from build123d import *

# Parameters (mm, degrees)
SZKIC1_R                    = 5
SZKIC1_R_2                  = 21.5
DODANIE_WYCI_GNI_CIE1_DEPTH = 3
DODANIE_WYCI_GNI_CIE2_DEPTH = 3


with BuildPart() as part:
    # Szkic1 → Dodanie-wyciągnięcie1 (new body)
    with BuildSketch(Plane.XY):
        with BuildLine():
            ThreePointArc((10, 35), (0, 45), (-10, 35))
            ThreePointArc((-10, 35), (-17.32233047, 17.32233047), (-35, 10))
            ThreePointArc((-35, 10), (-45, 0), (-35, -10))
            ThreePointArc((-35, -10), (-17.32233047, -17.32233047), (-10, -35))
            ThreePointArc((-10, -35), (0, -45), (10, -35))
            ThreePointArc((10, -35), (17.32233047, -17.32233047), (35, -10))
            ThreePointArc((35, -10), (45, 0), (35, 10))
            ThreePointArc((35, 10), (17.32233047, 17.32233047), (10, 35))
        make_face()
        with Locations((0, 35)):
            Circle(SZKIC1_R, mode=Mode.SUBTRACT)
        Circle(SZKIC1_R_2, mode=Mode.SUBTRACT)
        with Locations((35, 0)):
            Circle(SZKIC1_R, mode=Mode.SUBTRACT)
        with Locations((0, -35)):
            Circle(SZKIC1_R, mode=Mode.SUBTRACT)
        with Locations((-35, 0)):
            Circle(SZKIC1_R, mode=Mode.SUBTRACT)
    extrude(amount=DODANIE_WYCI_GNI_CIE1_DEPTH)

    # Szkic2 → Dodanie-wyciągnięcie2 (add)
    with BuildSketch(Plane.XY):
        with BuildLine():
            Line((27.599747415, 5.722247038), (37.016747674, 9.794525452))
            ThreePointArc((37.016747674, 9.794525452), (19.32662719, 19.32662719), (9.794525452, 37.016747674))
            Line((9.794525452, 37.016747674), (8.161162093, 24.785340239))
            Line((8.161162093, 24.785340239), (27.599747415, 5.722247038))
        make_face()
        with BuildLine():
            Line((-5.468778256, 25.979107706), (-9.794525452, 37.016747674))
            ThreePointArc((-9.794525452, 37.016747674), (-19.32662719, 19.32662719), (-37.016747674, 9.794525452))
            Line((-37.016747674, 9.794525452), (-28.775607604, 5.722247038))
            Line((-28.775607604, 5.722247038), (-5.468778256, 25.979107706))
        make_face()
        with BuildLine():
            ThreePointArc((-9.794525452, -37.016747674), (-19.32662719, -19.32662719), (-37.016747674, -9.794525452))
            Line((-37.016747674, -9.794525452), (-27.727906649, -4.880240326))
            Line((-27.727906649, -4.880240326), (-6.103941432, -26.086498779))
            Line((-6.103941432, -26.086498779), (-9.794525452, -37.016747674))
        make_face()
        with BuildLine():
            ThreePointArc((9.794525452, -37.016747674), (19.32662719, -19.32662719), (37.016747674, -9.794525452))
            Line((37.016747674, -9.794525452), (25.012487301, -7.237711123))
            Line((25.012487301, -7.237711123), (6.527798735, -26.086498779))
            Line((6.527798735, -26.086498779), (9.794525452, -37.016747674))
        make_face()
    extrude(amount=DODANIE_WYCI_GNI_CIE2_DEPTH)


solid = part.part
Here's how the part is built. I have some questions about the finished solid (model axes, mm). Round coordinates to 2 decimals unless told otherwise and drop trailing zeros. Order: outer loops, then holes, each group sorted by start corner. A loop starts at its lowest first (then second) coordinate and runs counter-clockwise, first axis right, second up. Notation, with made-up numbers: M 23,35.5 L 42,35.5 A25 cw 42,59.5 Z; hole C -4.75,-13.75 d3. An arc over 180 degrees is marked long. Return JSON: item names as keys, results as strings. Group by question number.
1. Please list where these lines run through material, in increasing order: probe 1 along Y at (x, z) = (1.5, 0.3); probe 2 along X at (y, z) = (39, 1.85); probe 3 along X at (y, z) = (5.5, 0.95).
2. If we section it at C-C on z = 0.75: List the corners of the cut face in (x, y) for me, then the cut area to 3 significant figures.
3. If we section it at A-A on x = 0: List the corners of the cut face in (y, z) for me, then the cut area to 3 significant figures.
4. If we section it at D-D on y = -32.5: List the corners of the cut face in (x, z) for me.
5. If we mould it in two halves opening along Y, with no side actions, what happens to faces 1 (the face through (30, 0, 1)), 2 (the face through (-45, 0, 1)), 3 (the face through (-19.126, -19.529, 1.479))? For each: pulls with the +Y half, pulls with the -Y half, needs draft (parallel to the pull), parting line crosses it, or undercut.
6. I'm going to push flat-ended pins straight in: pin 1 Ø16 at (x, y) = (35, 0) entering from -Z; pin 2 Ø6 at (x, y) = (-35, 0) entering from -Z. Where does each tip first touch, or does it pass through?
Reply:
{
 "1": {"probe 1": "-44.89 to -39.77, -30.23 to -21.45, 21.45 to 30.23, 39.77 to 44.89", "probe 2": "-9.17 to -3, 3 to 9.17", "probe 3": "-43.35 to -20.78, 20.78 to 43.35"},
 "2": {"outline": "M -37.02,-9.79 A35 cw -9.79,-37.02 A10 ccw 9.79,-37.02 A35 cw 37.02,-9.79 A10 ccw 37.02,9.79 A35 cw 9.79,37.02 A10 ccw -9.79,37.02 A35 cw -37.02,9.79 A10 ccw Z; hole C -35,0 d10; hole C 0,0 d43; hole C 0,-35 d10; hole C 0,35 d10; hole C 35,0 d10", "area": "2,100 mm^2"},
 "3": {"outline": "M -45,0 L -40,0 L -40,3 L -45,3 Z; M -30,0 L -21.5,0 L -21.5,3 L -30,3 Z; M 21.5,0 L 30,0 L 30,3 L 21.5,3 Z; M 40,0 L 45,0 L 45,3 L 40,3 Z", "area": "81.0 mm^2"},
 "4": {"outline": "M -11.04,0 L -4.33,0 L -4.33,3 L -11.04,3 Z; M 4.33,0 L 11.04,0 L 11.04,3 L 4.33,3 Z"},
 "5": {"face 1": "undercut", "face 2": "parting line crosses it", "face 3": "pulls with the -Y half"},
 "6": {"pin 1": "z = 0", "pin 2": "through"}
}
